```python
from build123d import *

# Parameters (mm, degrees)
SCHIZZO3_R                   = 1.5
ESTRUSIONE_ESTRUSIONE1_DEPTH = 5
SCHIZZO2_R                   = 2
SCHIZZO2_R_2                 = 12.5
SCHIZZO2_R_3                 = 1.5
TAGLIO_ESTRUSIONE1_DEPTH     = 6
TAGLIO_ESTRUSIONE2_DEPTH     = 6
SCHIZZO6_R                   = 1.5
SCHIZZO6_R_2                 = 4
SCHIZZO6_W                   = 5
SCHIZZO6_H                   = 12.5
TAGLIO_ESTRUSIONE4_DEPTH     = 6


with BuildPart() as part:
    # Schizzo3 → Estrusione-Estrusione1 (new body)
    with BuildSketch(Plane(origin=(0, 0, 0), x_dir=(0, 0, -1), z_dir=(1, 0, 0))):
        with BuildLine():
            Line((-95, -33), (201, -33))
            ThreePointArc((201, -33), (233.396512744, -6.282194046), (213.334616938, 30.608123513))
            Line((213.334616938, 30.608123513), (12.334616938, 111.608123513))
            ThreePointArc((12.334616938, 111.608123513), (-5.305430843, 113.570729245), (-21.410737295, 106.111358555))
            Line((-21.410737295, 106.111358555), (-116.410737295, 25.111358555))
            ThreePointArc((-116.410737295, 25.111358555), (-125.96509997, -11.408881796), (-95, -33))
        make_face()
        with Locations((-65.666686189, 61.806607259)):
            Circle(SCHIZZO3_R, mode=Mode.SUBTRACT)
        with Locations((110.965735584, 66.470529041)):
            Circle(SCHIZZO3_R, mode=Mode.SUBTRACT)
        with Locations((73.86497981, 81.421579875)):
            Circle(SCHIZZO3_R, mode=Mode.SUBTRACT)
        with Locations((148.066491357, 51.519478207)):
            Circle(SCHIZZO3_R, mode=Mode.SUBTRACT)
    extrude(amount=ESTRUSIONE_ESTRUSIONE1_DEPTH)

    # Schizzo2 → Taglio-Estrusione1 (cut, through all)
    with BuildSketch(Plane(origin=(0, 0, 0), x_dir=(0, 0, -1), z_dir=(1, 0, 0))):
        with Locations((-95, 0)):
            Circle(SCHIZZO2_R)
        with Locations((201, 0)):
            Circle(SCHIZZO2_R)
        with Locations((0, 81)):
            Circle(SCHIZZO2_R_2)
        with Locations((0, 101)):
            Circle(SCHIZZO2_R_3)
        with Locations((20, 81)):
            Circle(SCHIZZO2_R_3)
        with Locations((-20, 81)):
            Circle(SCHIZZO2_R_3)
        with Locations((0, 61)):
            Circle(SCHIZZO2_R_3)
    extrude(amount=TAGLIO_ESTRUSIONE1_DEPTH, mode=Mode.SUBTRACT)

    # Schizzo4 → Taglio-Estrusione2 (cut, through all)
    with BuildSketch(Plane(origin=(0, 0, 0), x_dir=(0, 0, -1), z_dir=(1, 0, 0))):
        Polygon((104.943784553, 71.592648309), (103.074903199, 66.955053837), (79.886930841, 76.299460608), (81.755812195, 80.93705508), align=None)
        Polygon((118.856567968, 65.986004246), (116.987686614, 61.348409774), (140.175658973, 52.004003003), (142.044540327, 56.641597475), align=None)
        Polygon((-82.507716927, 50.732778486), (-72.995838686, 58.842906249), (-69.751787581, 55.038154953), (-79.263665822, 46.92802719), align=None)
        Polygon((-61.581584798, 68.575059565), (-58.337533692, 64.770308269), (-48.825655452, 72.880436032), (-52.069706557, 76.685187328), align=None)
    extrude(amount=TAGLIO_ESTRUSIONE2_DEPTH, mode=Mode.SUBTRACT)

    # Schizzo6 → Taglio-Estrusione4 (cut, through all)
    with BuildSketch(Plane(origin=(0, 0, 0), x_dir=(0, 0, -1), z_dir=(1, 0, 0))):
        with Locations((-95, 7)):
            Circle(SCHIZZO6_R)
        with Locations((-90, 7)):
            Circle(SCHIZZO6_R)
        with Locations((-85, 7)):
            Circle(SCHIZZO6_R)
        with Locations((-80, 7)):
            Circle(SCHIZZO6_R)
        with Locations((53, -15)):
            Circle(SCHIZZO6_R_2)
        with Locations((53, 20.84)):
            Circle(SCHIZZO6_R)
        with Locations((-100, 7)):
            Circle(SCHIZZO6_R)
        with Locations((-105, 7)):
            Circle(SCHIZZO6_R)
        with Locations((-110, 7)):
            Circle(SCHIZZO6_R)
        with Locations((-80, -7)):
            Circle(SCHIZZO6_R)
        with Locations((-85, -7)):
            Circle(SCHIZZO6_R)
        with Locations((-90, -7)):
            Circle(SCHIZZO6_R)
        with Locations((-95, -7)):
            Circle(SCHIZZO6_R)
        with Locations((-100, -7)):
            Circle(SCHIZZO6_R)
        with Locations((-105, -7)):
            Circle(SCHIZZO6_R)
        with Locations((-110, -7)):
            Circle(SCHIZZO6_R)
        with Locations((216, -7)):
            Circle(SCHIZZO6_R)
        with Locations((211, -7)):
            Circle(SCHIZZO6_R)
        with Locations((206, -7)):
            Circle(SCHIZZO6_R)
        with Locations((201, -7)):
            Circle(SCHIZZO6_R)
        with Locations((196, -7)):
            Circle(SCHIZZO6_R)
        with Locations((191, -7)):
            Circle(SCHIZZO6_R)
        with Locations((186, -7)):
            Circle(SCHIZZO6_R)
        with Locations((186, 7)):
            Circle(SCHIZZO6_R)
        with Locations((191, 7)):
            Circle(SCHIZZO6_R)
        with Locations((196, 7)):
            Circle(SCHIZZO6_R)
        with Locations((201, 7)):
            Circle(SCHIZZO6_R)
        with Locations((206, 7)):
            Circle(SCHIZZO6_R)
        with Locations((211, 7)):
            Circle(SCHIZZO6_R)
        with Locations((216, 7)):
            Circle(SCHIZZO6_R)
        with BuildLine():
            Line((-105, 2), (-85, 2))
            ThreePointArc((-85, 2), (-83, 0), (-85, -2))
            Line((-85, -2), (-105, -2))
            ThreePointArc((-105, -2), (-107, 0), (-105, 2))
        make_face()
        with BuildLine():
            Line((191, 2), (211, 2))
            ThreePointArc((211, 2), (213, 0), (211, -2))
            Line((211, -2), (191, -2))
            ThreePointArc((191, -2), (189, 0), (191, 2))
        make_face()
        with Locations((53, 34.59)):
            Rectangle(SCHIZZO6_W, SCHIZZO6_H)
        with Locations((53, 7.09)):
            Rectangle(SCHIZZO6_W, SCHIZZO6_H)
    extrude(amount=TAGLIO_ESTRUSIONE4_DEPTH, mode=Mode.SUBTRACT)


solid = part.part
```
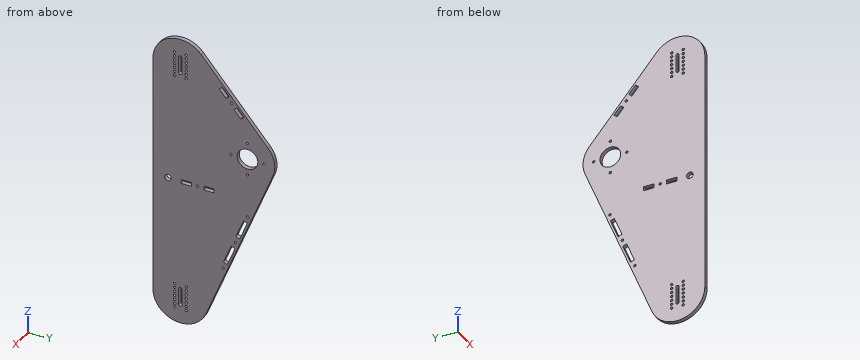
Read the model definition and answer for the solid it produces. Units are mm, in the model's axes. Coordinates: 2 decimals unless noted, no trailing zeros. Loops run counter-clockwise (first coordinate to the right, second up) from the corner with the lowest first, then second, coordinate; pieces in that order, holes last. Notation, with made-up numbers: (48, 58.5) -> (83, 58.5) arc R17 ccw to (83, 82.5) -> close; hole circle Ø6 at (84.5, 69). An arc over 180 degrees is marked (long way). Return JSON: item names as keys, results as strings.
Item 1: Find section C-C (z = 32). Determine the outline of the cut face in (x, y), plus the area to 3 significant figures.
Answers:
{"outline": "(0, -33) -> (5, -33) -> (5, 97.08) -> (0, 97.08) -> close", "area": "650 mm2"}
Item 2: Find the intervals of material crossed by probe 1 along Y at (x, z) = (2.3, 106); probe 2 along Y at (x, z) = (0.9, -211); probe 3 along Y at (x, z) = (2.75, 110), in increasing order.
Answers:
{"probe 1": "y = -31.11 to -8.12, -5.88 to -1.73, 1.73 to 5.88, 8.12 to 33.99", "probe 2": "y = -31.45 to -8.5, -5.5 to -2, 2 to 5.5, 8.5 to 31.55", "probe 3": "y = -29.39 to -8.5, -5.5 to 5.5, 8.5 to 30.58"}
Item 3: Find section A-A (z = -90). Determine the outline of the cut face in (x, y).
Answers:
{"outline": "(0, -33) -> (5, -33) -> (5, 72.22) -> (0, 72.22) -> close; (0, 77.61) -> (5, 77.61) -> (5, 80.31) -> (0, 80.31) -> close"}
Item 4: Find section B-B (x = 3). Count the separate pieces of the cut face and the enclosed holes in it, plus the area to 3 significant figures.
Answers:
{"separate pieces": "1", "enclosed holes": "47", "area": "35,000 mm2"}
Item 5: Flat-ended cylindrical pins translate along their axes: P1, Ø6, axis at y = -5.5, z = -116.5, coming from the -X side; P2, Ø1.5, axis at x = 1.5, y = 32, coming from the -Z side; P3, Ø1.5, axis at x = 1.5, y = 70.5, coming from the +Z side; P4, Ø3, axis at x = 3, y = -12.5, coming from the -Z side. Find the tip coordinate at first contact, or state that the pin passes through.
Answers:
{"P1": "stops at x = 0", "P2": "stops at z = -211.74", "P3": "stops at z = 64.06", "P4": "stops at z = -232.11"}
